```python
from build123d import *

# Parameters (mm, degrees)
SKETCH1_W                = 69.85
SKETCH1_H                = 57.15
BOSS_EXTRUDE1_DEPTH      = 15.24
SKETCH2_W                = 50.8
SKETCH2_H                = 6.35
CUT_EXTRUDE1_DEPTH       = 69.85
SKETCH3_W                = 44.45
SKETCH3_H                = 4.826
CUT_EXTRUDE2_DEPTH       = 50.8
SKETCH5_W                = 61.722
SKETCH5_H                = 20.0000108
SKETCH5_R                = 0.81915
CUT_EXTRUDE3_DEPTH       = 1.016
SKETCH5_3_R              = 0.81915
CUT_EXTRUDE4_DEPTH       = 16.24
SKETCH7_W                = 69.85
SKETCH7_H                = 6.096
BOSS_EXTRUDE2_DEPTH      = 6.35
SKETCH8_W                = 6.35
SKETCH8_H                = 1.27
CUT_EXTRUDE9_DEPTH       = 1
CUT_EXTRUDE9_DEPTH_BACK  = 70.85
SKETCH17_W               = 22.225
SKETCH17_H               = 4.826
CUT_EXTRUDE13_DEPTH      = 6.35
SKETCH18_W               = 22.225
SKETCH18_H               = 29.21
CUT_EXTRUDE14_DEPTH      = 1
CUT_EXTRUDE14_DEPTH_BACK = 16.24
FILLET1_R                = 2.54
SKETCH19_W               = 30.48
SKETCH19_H               = 33.3399892
CUT_EXTRUDE16_DEPTH      = 1.016


with BuildPart() as part:
    # Sketch1 → Boss-Extrude1 (new body)
    with BuildSketch(Plane(origin=(0, 0, 0), x_dir=(1, 0, 0), z_dir=(0, 1, 0))):
        Rectangle(SKETCH1_W, SKETCH1_H)
    extrude(amount=BOSS_EXTRUDE1_DEPTH)

    # Sketch2 → Cut-Extrude1 (cut)
    with BuildSketch(Plane.ZY.offset(34.925)):
        with Locations((-3.175, 7.239)):
            Rectangle(SKETCH2_W, SKETCH2_H)
    extrude(amount=-CUT_EXTRUDE1_DEPTH, mode=Mode.SUBTRACT)

    # Sketch3 → Cut-Extrude2 (cut)
    with BuildSketch(Plane.ZY.offset(34.925)):
        with Locations((-6.35, 12.827)):
            Rectangle(SKETCH3_W, SKETCH3_H)
    cut_extrude2 = extrude(amount=-CUT_EXTRUDE2_DEPTH, mode=Mode.SUBTRACT)

    # Mirror1: Cut-Extrude2 across plane
    add(cut_extrude2.mirror(Plane(origin=(0, 0, 0), x_dir=(0, 0, 1), z_dir=(1, 0, 0))), mode=Mode.SUBTRACT)

    # Sketch5 → Cut-Extrude3 (cut)
    with BuildSketch(Plane.XZ):
        with Locations((0, -14.7649946)):
            Rectangle(SKETCH5_W, SKETCH5_H)
        with Locations((-27.8892, -7.3049892)):
            Circle(SKETCH5_R, mode=Mode.SUBTRACT)
        with Locations((27.9908, -7.3049892)):
            Circle(SKETCH5_R, mode=Mode.SUBTRACT)
    extrude(amount=-CUT_EXTRUDE3_DEPTH, mode=Mode.SUBTRACT)

    # Sketch5<3> → Cut-Extrude4 (cut, through all)
    with BuildSketch(Plane.XZ):
        with Locations((-27.9908, -22.225)):
            Circle(SKETCH5_3_R)
        with Locations((27.9908, -22.225)):
            Circle(SKETCH5_3_R)
        with Locations((-27.8892, -7.3049892)):
            Circle(SKETCH5_3_R)
        with Locations((27.9908, -7.3049892)):
            Circle(SKETCH5_3_R)
    extrude(amount=-CUT_EXTRUDE4_DEPTH, mode=Mode.SUBTRACT)

    # Sketch7 → Boss-Extrude2 (add)
    with BuildSketch(Plane(origin=(0, 0, 22.225), x_dir=(-1, 0, 0), z_dir=(0, 0, -1))):
        with Locations((0, 12.192)):
            Rectangle(SKETCH7_W, SKETCH7_H)
    extrude(amount=BOSS_EXTRUDE2_DEPTH)

    # Sketch8 → Cut-Extrude9 (cut, two sides)
    with BuildSketch(Plane.ZY.offset(34.925)) as cut_extrude9_sk:
        with Locations((19.05, 9.779)):
            Rectangle(SKETCH8_W, SKETCH8_H)
    extrude(amount=CUT_EXTRUDE9_DEPTH, mode=Mode.SUBTRACT)
    extrude(cut_extrude9_sk.sketch, amount=-CUT_EXTRUDE9_DEPTH_BACK, mode=Mode.SUBTRACT)

    # Sketch17 → Cut-Extrude13 (cut)
    with BuildSketch(Plane(origin=(0, 0, 15.875), x_dir=(-1, 0, 0), z_dir=(0, 0, -1))):
        with Locations((-23.8125, 12.827)):
            Rectangle(SKETCH17_W, SKETCH17_H)
        with Locations((23.8125, 12.827)):
            Rectangle(SKETCH17_W, SKETCH17_H)
    extrude(amount=-CUT_EXTRUDE13_DEPTH, mode=Mode.SUBTRACT)

    # Sketch18 → Cut-Extrude14 (cut, two sides)
    with BuildSketch(Plane(origin=(0, 15.24, 0), x_dir=(1, 0, 0), z_dir=(0, 1, 0))) as cut_extrude14_sk:
        with Locations((-23.8125, -13.97)):
            Rectangle(SKETCH18_W, SKETCH18_H)
        with Locations((23.8125, -13.97)):
            Rectangle(SKETCH18_W, SKETCH18_H)
    extrude(amount=CUT_EXTRUDE14_DEPTH, mode=Mode.SUBTRACT)
    extrude(cut_extrude14_sk.sketch, amount=-CUT_EXTRUDE14_DEPTH_BACK, mode=Mode.SUBTRACT)

    # Fillet1
    fillet1_edges = [part.edges().sort_by_distance(p)[0] for p in [
        (-34.925, 2.032, -28.575),
        (34.925, 2.032, -28.575),
        (-34.925, 2.032, -0.635),
        (-12.7, 2.032, -0.635),
        (34.925, 2.032, -0.635),
        (12.7, 2.032, -0.635),
    ]]
    fillet(fillet1_edges, radius=FILLET1_R)

    # Sketch19 → Cut-Extrude16 (cut)
    with BuildSketch(Plane.XZ):
        with Locations((0, 11.9050054)):
            Rectangle(SKETCH19_W, SKETCH19_H)
    extrude(amount=-CUT_EXTRUDE16_DEPTH, mode=Mode.SUBTRACT)


solid = part.part
```
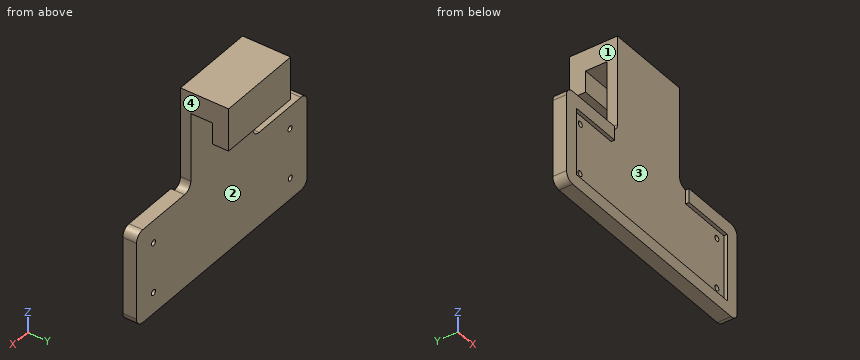
Design review of the part built by this model. Coordinates are the model's own, in mm. Face numbers are marked on the shaded views. Coordinates: 2 decimals unless noted, no trailing zeros. Order: outer loops, then holes, each group sorted by start corner. A loop starts at its lowest first (then second) coordinate and runs counter-clockwise, first axis right, second up.
1) Take a section at A-A, the plane z = 20.5. Give the boundary of the cut face in (x, y), and give its area (3 significant figures).
2) Wall thickness on line 1 along Z through (x, y) = (-23, 2.25) (3 decimals); line 2 along Y through (x, z) = (-1.5, -3.5); line 3 along Z through (x, y) = (4.5, 11.25) (3 decimals): over which ranges is each line inside the solid? List them lowest first.
3) Take a section at D-D, the plane y = 1.75. Give the boundary of the cut face in (x, z) (3 decimals).
4) Clearance check with flat-ended pins moving along their axes: pin 1 (5 mm diameter, centred on x = -0.5, y = 6.5, fed in from -Z) (3 decimals); pin 2 (1.5 mm diameter, centred on x = -18.5, y = 3.5, fed in from +Z) (3 decimals); pin 3 (3 mm diameter, centred on x = -5.5, z = 18, fed in from -Y); pin 4 (7 mm diameter, centred on y = 11, z = 19, fed in from +X). State where each tip first meets the part, or that it passes through.
5) Take a section at B-B, the plane x = 18. Give the boundary of the cut face in (y, z) (3 decimals).
6) Mouldability with a two-part tool opening along X and no side actions: class the marked faces 1, 2, 3 and 4 as +X half, -X half, draft (parallel to the pull), parting line (faces both ways), or undercut.
7) Take a section at C-C, the plane z = -12.5. Give the boundary of the cut face in (x, y) (3 decimals), and give its area (3 significant figures).
Returned:
1. outline: (-12.7, 1.02) - (12.7, 1.02) - (12.7, 4.06) - (-12.7, 4.06) - close; (-12.7, 10.41) - (12.7, 10.41) - (12.7, 15.24) - (-12.7, 15.24) - close
1. area: 200 mm2
2. line 1: z = -28.575 to -0.635
2. line 2: y = 1.02 to 4.06
2. line 3: z = 15.875 to 28.575
3. outline: (-34.925, -26.035) arc R2.54 ccw to (-32.385, -28.575) - (32.385, -28.575) arc R2.54 ccw to (34.925, -26.035) - (34.925, -3.175) arc R2.54 ccw to (32.385, -0.635) - (15.24, -0.635) arc R2.54 cw to (12.7, 1.905) - (12.7, 28.575) - (-12.7, 28.575) - (-12.7, 1.905) arc R2.54 cw to (-15.24, -0.635) - (-32.385, -0.635) arc R2.54 ccw to (-34.925, -3.175) - close; hole circle Ø1.638 at (-27.991, -22.225); hole circle Ø1.638 at (-27.889, -7.305); hole circle Ø1.638 at (27.991, -22.225); hole circle Ø1.638 at (27.991, -7.305)
4. pin 1: stops at z = -28.575
4. pin 2: stops at z = -0.635
4. pin 3: stops at y = 1.02
4. pin 4: stops at x = 12.7
5. outline: (0, -28.575) - (4.064, -28.575) - (4.064, -0.635) - (0, -0.635) - (0, -4.765) - (1.016, -4.765) - (1.016, -24.765) - (0, -24.765) - close
6. face 1: -X half
6. face 2: draft
6. face 3: undercut
6. face 4: +X half
7. outline: (-34.925, 0) - (-30.861, 0) - (-30.861, 1.016) - (30.861, 1.016) - (30.861, 0) - (34.925, 0) - (34.925, 4.064) - (-34.925, 4.064) - close
7. area: 221 mm2
